Could you check a few things on this drawing? It's one solid part, dimensions in mm from its lowest x, y, z. Round coordinates to 2 decimals unless told otherwise and drop trailing zeros. Order: outer loops, then holes, each group sorted by start corner. A loop starts at its lowest first (then second) coordinate and runs counter-clockwise, first axis right, second up. Notation, with made-up numbers: (-31.5, 12.25) - (-10.5, 12.25) arc R26 cw to (-10.5, 30.25) - close; hole circle Ø2 at (7, 17.25). An arc over 180 degrees is marked (long way). Use one line per item in the form item = value.
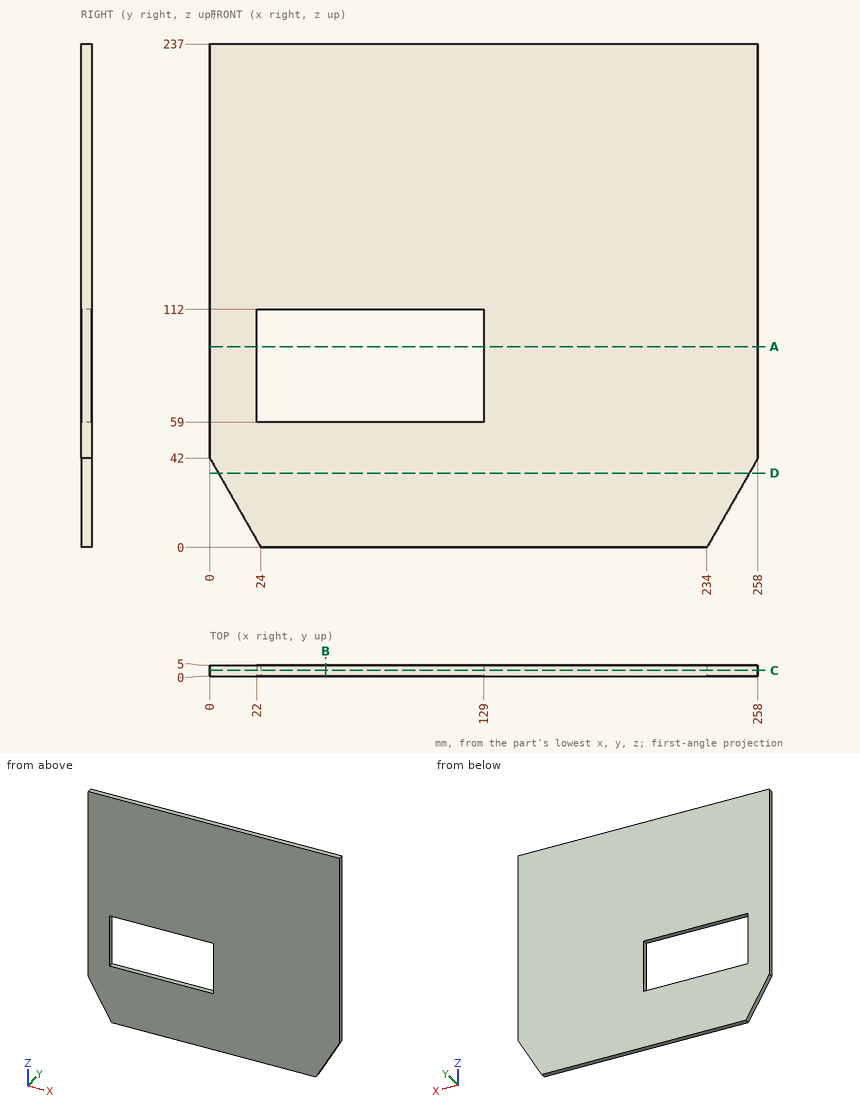
Item 1: Imagine slicing it at D-D on z = 35. Please give me the cut outline in (x, y).
Found:
outline = (4, 0) - (254, 0) - (254, 5) - (4, 5) - close
Item 2: Imagine slicing it at A-A on z = 94.5. Please give me the cut outline in (x, y), plus the area to 3 significant figures.
Found:
outline = (0, 0) - (22, 0) - (22, 5) - (0, 5) - close; (129, 0) - (258, 0) - (258, 5) - (129, 5) - close
area = 755 mm2
Item 3: Will this pin go through, and if not, where does the flat tip stop? P1, Ø10, axis at x = 119, z = 131.5, coming from the -Y side.
Found:
P1 = 0
Item 4: Imagine slicing it at C-C on y = 2.7. Please give me the cut outline in (x, z), plus the area to 3 significant figures.
Found:
outline = (0, 42) - (24, 0) - (234, 0) - (258, 42) - (258, 237) - (0, 237) - close; hole (22, 59) - (129, 59) - (129, 112) - (22, 112) - close
area = 54,500 mm2
Item 5: Imagine slicing it at B-B on x = 54.5. Please give me the cut outline in (y, z).
Found:
outline = (0, 0) - (5, 0) - (5, 59) - (0, 59) - close; (0, 112) - (5, 112) - (5, 237) - (0, 237) - close
Item 6: I need wall thicknesses on L1, parallel to X at y = 1.6, z = 106; L2, parallel to Z at x = 120, y = 0.35; L3, parallel to Z at x = 12.5, y = 3.65 (3 decimals). Which ranges of each line are inside material? Lowest first, please.
Found:
L1 = 0 to 22, 129 to 258
L2 = 0 to 59, 112 to 237
L3 = 20.125 to 237
